from build123d import *

# Parameters (mm, degrees)
SKETCH1_R           = 27.94
BOSS_EXTRUDE1_DEPTH = 25.89
CUT_EXTRUDE2_DEPTH  = 48.239594621
SKETCH4_R           = 4.5
SKETCH4_R_2         = 2
BOSS_EXTRUDE3_DEPTH = 7


with BuildPart() as part:
    # Sketch1 → Boss-Extrude1 (new body)
    with BuildSketch(Plane(origin=(0, 0, 0), x_dir=(1, 0, 0), z_dir=(0, 1, 0))):
        with Locations(Location((0, 0, 0), (0, 0, 270))):
            Circle(SKETCH1_R)
    extrude(amount=BOSS_EXTRUDE1_DEPTH)

    # Sketch2 → Cut-Extrude2 (cut, through all)
    with BuildSketch(Plane.XZ):
        with BuildLine():
            Line((1.479590886, 8.877545314), (3.342404051, 20.054424305))
            ThreePointArc((3.342404051, 20.054424305), (0, 24), (-3.342404051, 20.054424305))
            Line((-3.342404051, 20.054424305), (-1.479590886, 8.877545314))
            ThreePointArc((-1.479590886, 8.877545314), (0, 7.624143795), (1.479590886, 8.877545314))
        make_face()
        with BuildLine():
            Line((7.323601241, 5.231143743), (16.544055988, 11.817182849))
            ThreePointArc((16.544055988, 11.817182849), (16.970562748, 16.970562748), (11.817182849, 16.544055988))
            Line((11.817182849, 16.544055988), (5.231143743, 7.323601241))
            ThreePointArc((5.231143743, 7.323601241), (5.391083779, 5.391083779), (7.323601241, 5.231143743))
        make_face()
        with BuildLine():
            Line((8.877545314, -1.479590886), (20.054424305, -3.342404051))
            ThreePointArc((20.054424305, -3.342404051), (24, 0), (20.054424305, 3.342404051))
            Line((20.054424305, 3.342404051), (8.877545314, 1.479590886))
            ThreePointArc((8.877545314, 1.479590886), (7.624143795, 0), (8.877545314, -1.479590886))
        make_face()
        with BuildLine():
            Line((5.231143743, -7.323601241), (11.817182849, -16.544055988))
            ThreePointArc((11.817182849, -16.544055988), (16.970562748, -16.970562748), (16.544055988, -11.817182849))
            Line((16.544055988, -11.817182849), (7.323601241, -5.231143743))
            ThreePointArc((7.323601241, -5.231143743), (5.391083779, -5.391083779), (5.231143743, -7.323601241))
        make_face()
        with BuildLine():
            Line((-1.479590886, -8.877545314), (-3.342404051, -20.054424305))
            ThreePointArc((-3.342404051, -20.054424305), (0, -24), (3.342404051, -20.054424305))
            Line((3.342404051, -20.054424305), (1.479590886, -8.877545314))
            ThreePointArc((1.479590886, -8.877545314), (0, -7.624143795), (-1.479590886, -8.877545314))
        make_face()
        with BuildLine():
            Line((-7.323601241, -5.231143743), (-16.544055988, -11.817182849))
            ThreePointArc((-16.544055988, -11.817182849), (-16.970562748, -16.970562748), (-11.817182849, -16.544055988))
            Line((-11.817182849, -16.544055988), (-5.231143743, -7.323601241))
            ThreePointArc((-5.231143743, -7.323601241), (-5.391083779, -5.391083779), (-7.323601241, -5.231143743))
        make_face()
        with BuildLine():
            Line((-8.877545314, 1.479590886), (-20.054424305, 3.342404051))
            ThreePointArc((-20.054424305, 3.342404051), (-24, 0), (-20.054424305, -3.342404051))
            Line((-20.054424305, -3.342404051), (-8.877545314, -1.479590886))
            ThreePointArc((-8.877545314, -1.479590886), (-7.624143795, 0), (-8.877545314, 1.479590886))
        make_face()
        with BuildLine():
            Line((-5.231143743, 7.323601241), (-11.817182849, 16.544055988))
            ThreePointArc((-11.817182849, 16.544055988), (-16.970562748, 16.970562748), (-16.544055988, 11.817182849))
            Line((-16.544055988, 11.817182849), (-7.323601241, 5.231143743))
            ThreePointArc((-7.323601241, 5.231143743), (-5.391083779, 5.391083779), (-5.231143743, 7.323601241))
        make_face()
    extrude(amount=-CUT_EXTRUDE2_DEPTH, mode=Mode.SUBTRACT)

    # Sketch4 → Boss-Extrude3 (add)
    with BuildSketch(Plane(origin=(0, 0, 0), x_dir=(-1, 0, 0), z_dir=(0, -1, 0))):
        with Locations(Location((0, 0, 0), (0, 0, 270))):
            Circle(SKETCH4_R)
        with Locations(Location((0, 0, 0), (0, 0, 90))):
            Circle(SKETCH4_R_2, mode=Mode.SUBTRACT)
    extrude(amount=BOSS_EXTRUDE3_DEPTH)


solid = part.part
CAD build for the part. Positions are in the model's coordinates, mm. A direction names the side the tool comes from. Coordinates: 2 decimals unless noted, no trailing zeros. Loops run counter-clockwise (first coordinate to the right, second up) from the corner with the lowest first, then second, coordinate; pieces in that order, holes last. Notation, with made-up numbers: (-15.5, 35) -> (-6.5, 35) arc R26 cw to (-6.5, 57) -> close; hole circle Ø6 at (-5.5, 37.5). An arc over 180 degrees is marked (long way). One line per item, written item: value.
1. Pull direction X, two halves, no side cores. Call faces 1 (the face through (14.544, 12.764, 2.424)), 2 (the face through (1, -7, 2)): pulls with the +X half, pulls with the -X half, needs draft (parallel to the pull), parting line crosses it, or undercut.
Answers:
face 1: undercut
face 2: needs draft
2. Slice it at A-A on y = 13. Give the number of separate pieces and of enclosed holes in the cut face, and give its area (3 significant figures).
Answers:
separate pieces: 1
enclosed holes: 8
area: 1,820 mm^2
3. Which spindle directions (+Z, -Z, +X, -X, +Y, -Y) get a long thin tool onto all of the face, cutting with end or side? Do faces 3 (the face through (0, 25.89, 0)), 4 (the face through (2.4, 12.8, 14.4)), 5 (the face through (-2, -3, 0)). Say none if no direction does.
Answers:
face 3: +Z, -Z, +X, -X, +Y
face 4: +Y, -Y
face 5: -Y
4. Flat gauge pins, fed straight in: P1, Ø1.5, axis at y = 6, z = -10.5, coming from the -X side; P2, Ø5, axis at x = 21.5, z = -3.5, coming from the -Y side; P3, Ø5, axis at y = 18, z = -10.5, coming from the +X side. Where does each tip first touch, or does it go through?
Answers:
P1: stops at x = -26.18
P2: stops at y = 0
P3: stops at x = 26.77
5. Slice it at B-B on z = 0. Write the cut outline in (x, y).
Answers:
outline: (-27.94, 0) -> (-24, 0) -> (-24, 25.89) -> (-27.94, 25.89) -> close; (-7.62, 0) -> (-4.5, 0) -> (-4.5, -7) -> (-2, -7) -> (-2, 0) -> (2, 0) -> (2, -7) -> (4.5, -7) -> (4.5, 0) -> (7.62, 0) -> (7.62, 25.89) -> (-7.62, 25.89) -> close; (24, 0) -> (27.94, 0) -> (27.94, 25.89) -> (24, 25.89) -> close
6. Slice it at C-C on x = 0. Write the cut outline in (y, z).
Answers:
outline: (-7, -4.5) -> (0, -4.5) -> (0, -7.62) -> (25.89, -7.62) -> (25.89, 7.62) -> (0, 7.62) -> (0, 4.5) -> (-7, 4.5) -> (-7, 2) -> (0, 2) -> (0, -2) -> (-7, -2) -> close; (0, -27.94) -> (25.89, -27.94) -> (25.89, -24) -> (0, -24) -> close; (0, 24) -> (25.89, 24) -> (25.89, 27.94) -> (0, 27.94) -> close
7. Drill centre lines: line 1 (X direction, y = 6, z = -13.5); line 2 (Z direction, x = -16.5, y = 25); line 3 (Z direction, x = -17, y = 10.5). Where is each one in solid material? Low to high. Write a range as [from, to].
Answers:
line 1: x = [-24.46, -17.79], [-9.64, -2.25], [2.25, 9.64], [17.79, 24.46]
line 2: z = [-22.55, -17.36], [-11.79, -2.75], [2.75, 11.79], [17.36, 22.55]
line 3: z = [-22.17, -16.94], [-12.21, -2.83], [2.83, 12.21], [16.94, 22.17]
8. Slice it at D-D on z = -22. Write the cut outline in (x, y).
Answers:
outline: (-17.22, 0) -> (-3.09, 0) -> (-3.09, 25.89) -> (-17.22, 25.89) -> close; (3.09, 0) -> (17.22, 0) -> (17.22, 25.89) -> (3.09, 25.89) -> close
